Geometry check sheet. Reference: the model listing, model coordinates, mm. Face numbers are marked on the shaded views. A direction names the side the tool comes from. Coordinates: 2 decimals unless noted, no trailing zeros. Write each loop counter-clockwise with the first axis right and the second up, starting at its lowest first coordinate (ties: lowest second). Pieces come first, ordered by that corner, then holes. Notation, with made-up numbers: (15, -4) -> (44, -4) arc R24 ccw to (44, 13) -> close; hole circle Ø2 at (60.5, -38). An arc over 180 degrees is marked (long way). Answer as CSV lines item,"result".
```python
from build123d import *

# Parameters (mm, degrees)
BOSS_EXTRUDE2_DEPTH                            = 34.6202
CBORE_FOR_8_SOCKET_HEAD_CAP_SCREW2_D           = 4.4958
CBORE_FOR_8_SOCKET_HEAD_CAP_SCREW2_CBORE_D     = 7.9375
CBORE_FOR_8_SOCKET_HEAD_CAP_SCREW2_CBORE_DEPTH = 23.2156
FILLET2_R                                      = 4.55168
FILLET3_R                                      = 2.54


with BuildPart() as part:
    # Sketch1 → Boss-Extrude2 (new body)
    with BuildSketch(Plane(origin=(0, 0, 0), x_dir=(1, 0, 0), z_dir=(0, 1, 0))):
        Polygon((45.13707, 35.2425), (-26.08707, 35.2425), (-26.08707, 22.5425), (26.08707, 22.5425), (26.08707, -22.5425), (-26.08707, -22.5425), (-26.08707, -35.2425), (45.13707, -35.2425), align=None)
    extrude(amount=BOSS_EXTRUDE2_DEPTH)

    # CBORE for #8 Socket Head Cap Screw2 (through all)
    with Locations(Plane(origin=(0, 34.6202, 0), x_dir=(1, 0, 0), z_dir=(0, 1, 0))):
        with Locations((-72.97293, 28.8925), (38.78707, 28.8925), (38.78707, -28.8925), (-72.97293, -28.8925), (-17.09293, 28.8925), (-17.09293, -28.8925)):
            CounterBoreHole(CBORE_FOR_8_SOCKET_HEAD_CAP_SCREW2_D / 2, CBORE_FOR_8_SOCKET_HEAD_CAP_SCREW2_CBORE_D / 2, CBORE_FOR_8_SOCKET_HEAD_CAP_SCREW2_CBORE_DEPTH)

    # Fillet2
    fillet2_edges = [part.edges().sort_by_distance(p)[0] for p in [
        (26.08707, 17.3101, 22.5425),
        (26.08707, 17.3101, -22.5425),
    ]]
    fillet(fillet2_edges, radius=FILLET2_R)

    # Fillet3
    fillet3_edges = [part.edges().sort_by_distance(p)[0] for p in [
        (45.13707, 17.3101, -35.2425),
        (45.13707, 17.3101, 35.2425),
        (-26.08707, 17.3101, 35.2425),
        (-26.08707, 17.3101, -35.2425),
    ]]
    fillet(fillet3_edges, radius=FILLET3_R)


solid = part.part
```
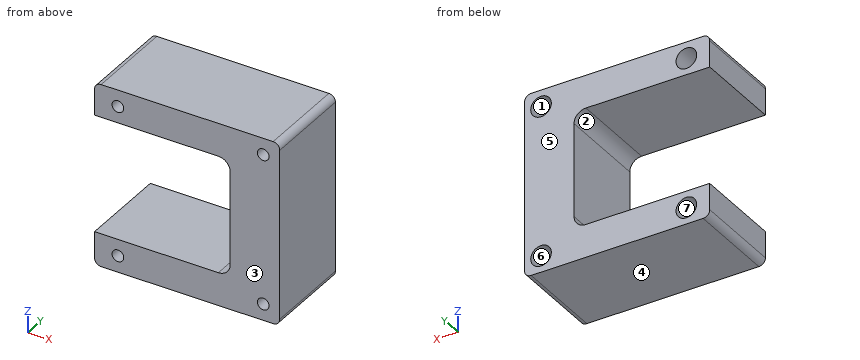
Item 1: Cross-section at A-A, the plane x = 15.5. Record the cut outline in (y, z).
Responses:
outline,"(0, -35.24) -> (34.62, -35.24) -> (34.62, -22.54) -> (0, -22.54) -> close; (0, 22.54) -> (34.62, 22.54) -> (34.62, 35.24) -> (0, 35.24) -> close"
Item 2: Cross-section at B-B, the plane y = 6.5. Record the cut outline in (x, z), plus the area to 3 significant figures.
Responses:
outline,"(-26.09, -32.7) arc R2.54 ccw to (-23.55, -35.24) -> (42.6, -35.24) arc R2.54 ccw to (45.14, -32.7) -> (45.14, 32.7) arc R2.54 ccw to (42.6, 35.24) -> (-23.55, 35.24) arc R2.54 ccw to (-26.09, 32.7) -> (-26.09, 22.54) -> (21.54, 22.54) arc R4.55 cw to (26.09, 17.99) -> (26.09, -17.99) arc R4.55 cw to (21.54, -22.54) -> (-26.09, -22.54) -> close; hole circle Ø4.5 at (-17.09, -28.89); hole circle Ø4.5 at (-17.09, 28.89); hole circle Ø4.5 at (38.79, -28.89); hole circle Ø4.5 at (38.79, 28.89)"
area,"2,610 mm2"
Item 3: Set-up check for the marked faces 1, 2 and 3: record each of +Z, -Z, +X, -X, +Y, -Y from which the full face is reachable in a straight line by a thin tool's end or side.
Responses:
face 1,"+Y"
face 2,"-X, +Y, -Y"
face 3,"+Z, -Z, +X, -X, -Y"
Item 4: Cross-section at C-C, the plane x = 23. Record the cut outline in (y, z), plus the area to 3 significant figures.
Responses:
outline,"(0, -35.24) -> (34.62, -35.24) -> (34.62, -22.3) -> (0, -22.3) -> close; (0, 22.3) -> (34.62, 22.3) -> (34.62, 35.24) -> (0, 35.24) -> close"
area,"896 mm2"
Item 5: Release check for a two-part mould opening along Z. For the marked faces 4, 5, 6 and 7 record: +Z half, -Z half, draft (parallel to the pull), parting line (faces both ways), or undercut.
Responses:
face 4,"-Z half"
face 5,"draft"
face 6,"undercut"
face 7,"undercut"
Item 6: Depth check by flat-ended pin: pin 1 Ø1 at (y, z) = (7, -21) entering from -X; pin 2 Ø6.5 at (x, z) = (-17.09, -28.89) entering from +Y; pin 3 Ø17.5 at (y, z) = (12.5, -3) entering from -X; pin 4 Ø2.5 at (x, z) = (38.79, 28.89) entering from +Y. Enter the tip coordinate at first touch or a pass-through.
Responses:
pin 1,"stops at x = 24.43"
pin 2,"stops at y = 11.4"
pin 3,"stops at x = 26.09"
pin 4,"passes through"
Item 7: Thickness scan on probe 1 along X at (y, z) = (11, 29); probe 2 along X at (y, z) = (12.5, -29); probe 3 along Z at (x, y) = (41, 20). Record the ranges inside material, lowest first.
Responses:
probe 1,"x = -26.09 to -19.34, -14.85 to 36.54, 41.03 to 45.14"
probe 2,"x = -26.09 to -21.06, -13.13 to 34.82, 42.75 to 45.14"
probe 3,"z = -35.24 to -32.19, -25.6 to 25.6, 32.19 to 35.24"
Item 8: Cross-section at D-D, the plane z = 10. Record the cut outline in (x, y).
Responses:
outline,"(26.09, 0) -> (45.14, 0) -> (45.14, 34.62) -> (26.09, 34.62) -> close"
